Source: CAD feature listing. Evaluate the final solid. Frame: model axes, mm. A direction names the side the tool comes from. Round coordinates to 2 decimals unless told otherwise and drop trailing zeros. Write each loop counter-clockwise with the first axis right and the second up, starting at its lowest first coordinate (ties: lowest second). Pieces come first, ordered by that corner, then holes.
```python
from build123d import *

# Parameters (mm, degrees)
SKETCH017_W     = 71.6
SKETCH017_H     = 59.6
SKETCH017_W_2   = 65
SKETCH017_H_2   = 53
PAD009_DEPTH    = 9
SKETCH015_W     = 69.6
SKETCH015_H     = 57.6
POCKET004_DEPTH = 2.3
SKETCH016_W     = 4
SKETCH016_H     = 5.483822
SKETCH016_H_2   = 6.120376
SKETCH016_H_3   = 8.800861
SKETCH016_H_4   = 6.480469
SKETCH016_W_2   = 4.596547
SKETCH016_H_5   = 4
SKETCH016_W_3   = 6.834637
SKETCH016_W_4   = 8.377245
SKETCH016_W_5   = 7.094059
POCKET006_DEPTH = 4


with BuildPart() as part:
    # Sketch017 → Pad009 (new body)
    with BuildSketch(Plane.XY):
        with Locations((32.5, 26.5)):
            Rectangle(SKETCH017_W, SKETCH017_H)
        with Locations((32.5, 26.5)):
            Rectangle(SKETCH017_W_2, SKETCH017_H_2, mode=Mode.SUBTRACT)
    extrude(amount=PAD009_DEPTH)

    # Sketch015 (on Face10 of Pad009) → Pocket004 (cut)
    with BuildSketch(Plane.XY.offset(9)):
        with Locations((32.5, 26.5)):
            Rectangle(SKETCH015_W, SKETCH015_H)
    extrude(amount=-POCKET004_DEPTH, mode=Mode.SUBTRACT)

    # Sketch016 (on Face5 of Pocket004) → Pocket006 (cut)
    with BuildSketch(Plane.XY.offset(9)):
        with Locations((12.880272, 55.392385)):
            Rectangle(SKETCH016_W, SKETCH016_H)
        with Locations((29.880272, 54.935013)):
            Rectangle(SKETCH016_W, SKETCH016_H_2)
        with Locations((46.880272, 55.440656)):
            Rectangle(SKETCH016_W, SKETCH016_H_3)
        with Locations((63.880272, 54.707588)):
            Rectangle(SKETCH016_W, SKETCH016_H_4)
        with Locations((66.550759, 42.929046)):
            Rectangle(SKETCH016_W_2, SKETCH016_H_5)
        with Locations((68.417426, 28.929046)):
            Rectangle(SKETCH016_W_3, SKETCH016_H_5)
        with Locations((68.143181, 14.929046)):
            Rectangle(SKETCH016_W_4, SKETCH016_H_5)
        with Locations((68.408536, 0.929046)):
            Rectangle(SKETCH016_W_5, SKETCH016_H_5)
    extrude(amount=-POCKET006_DEPTH, mode=Mode.SUBTRACT)


with BuildPart() as part_1:
    # Body003 placement: moved
    add(part.part.moved(Location((8, 6, -9))))


solid = part_1.part
```
Q1. Section query D-D, the plane x = 13. Output: boundary loops of the cut face in (y, z).
Q2. Set-up query: faces 4 (the face through (35.88, 61, -3)), 5 (the face through (63, 61.3, -1)), 6 (the face through (40, 6, -6)), 7 (the face through (75, 21, -4)). Return all of +Z, -Z, +X, -X, +Y, -Y with unobstructed straight access to the full face (end or side cutting, diameter ignored); none if empty.
Q3. Section query C-C, the plane x = 37. Output: boundary loops of the cut face in (y, z), and give its area (3 significant figures).
Q4. Section query A-A, the plane z = -5.25. Output: boundary loops of the cut face in (x, y), and give its area (3 significant figures).
Q5. Section query B-B, the plane y = 17.5. Output: boundary loops of the cut face in (x, z).
Q6. Line query: line 1 (X direction, y = 15.5, z = -7.75); line 2 (Y direction, x = 26, z = -2); line 3 (Y direction, x = 17, z = -7.25). Output: solid intervals per line, ascending.
Q7. Pin query (flat end, axial travel): P1, Ø0.8, axis at y = 35.5, z = -3, coming from the +X side; P2, Ø3.5, axis at x = 74.5, y = 49, coming from the +Z side; P3, Ø2.5, axis at y = 21.5, z = -1.5, coming from the +X side. Return the tip coordinate at first contact, or that it passes through.
Q8. Mould query, pull axis X, two halves, no side actions, for faces 1 (the face through (76.3, 32, -5)), 2 (the face through (75, 18.929, -3)), 3 (the face through (74, 38, -2.3)). Classes: pulls with the +X half, pulls with the -X half, needs draft (parallel to the pull), parting line crosses it, or undercut.
Filled in:
1. outline: (2.7, -9) - (6, -9) - (6, -2.3) - (3.7, -2.3) - (3.7, 0) - (2.7, 0) - close; (59, -9) - (62.3, -9) - (62.3, 0) - (61.3, 0) - (61.3, -2.3) - (59, -2.3) - close
2. face 4: +Z, +Y
2. face 5: +Z
2. face 6: +Z, -Z
2. face 7: +Z, +X
3. outline: (2.7, -9) - (6, -9) - (6, -2.3) - (3.7, -2.3) - (3.7, 0) - (2.7, 0) - close; (59, -9) - (62.3, -9) - (62.3, -4) - (59, -4) - close
3. area: 40.9 mm2
4. outline: (4.7, 2.7) - (76.3, 2.7) - (76.3, 62.3) - (4.7, 62.3) - close; hole (8, 6) - (73, 6) - (73, 59) - (8, 59) - close
4. area: 822 mm2
5. outline: (4.7, -9) - (8, -9) - (8, -2.3) - (5.7, -2.3) - (5.7, 0) - (4.7, 0) - close; (73, -9) - (76.3, -9) - (76.3, 0) - (75.3, 0) - (75.3, -2.3) - (73, -2.3) - close
6. line 1: x = 4.7 to 8, 73 to 76.3
6. line 2: y = 2.7 to 3.7, 61.3 to 62.3
6. line 3: y = 2.7 to 6, 59 to 62.3
7. P1: stops at x = 73
7. P2: stops at z = -4
7. P3: stops at x = 8
8. face 1: pulls with the +X half
8. face 2: needs draft
8. face 3: undercut
